from build123d import *

# Parameters (mm, degrees)
F1_DEPTH = 5


with BuildPart() as f1:
    # F0 (on Front) → F1 (new body)
    with BuildSketch(Plane.XZ):
        with BuildLine():
            ThreePointArc((0, -3), (2.12132, -2.12132), (3, 0))
            ThreePointArc((3, 0), (2.992298, 0.214837), (2.96923, 0.428571))
            ThreePointArc((2.96923, 0.428571), (0, 3), (-2.96923, 0.428571))
            ThreePointArc((-2.96923, 0.428571), (-2.267787, -1.963961), (0, -3))
        make_face()
        with BuildLine():
            ThreePointArc((-1.322876, -1.5), (-0.822876, 1.822876), (2, 0))
            ThreePointArc((2, 0), (1.822876, -0.822876), (1.322876, -1.5))
            ThreePointArc((1.322876, -1.5), (0, -2), (-1.322876, -1.5))
        make_face(mode=Mode.SUBTRACT)
        with BuildLine():
            ThreePointArc((2.96923, 0.428571), (2.992298, 0.214837), (3, 0))
            ThreePointArc((3, 0), (2.12132, -2.12132), (0, -3))
            ThreePointArc((0, -3), (2.618615, -3.976284), (3.958973, -6.428571))
            Line((3.958973, -6.428571), (2.96923, 0.428571))
        make_face()
        with BuildLine():
            ThreePointArc((-3.958973, -6.428571), (-2.618615, -3.976284), (0, -3))
            ThreePointArc((0, -3), (-2.267787, -1.963961), (-2.96923, 0.428571))
            Line((-2.96923, 0.428571), (-3.958973, -6.428571))
        make_face()
        with BuildLine():
            ThreePointArc((3.958973, -6.428571), (2.618615, -3.976284), (0, -3))
            ThreePointArc((0, -3), (-2.618615, -3.976284), (-3.958973, -6.428571))
            ThreePointArc((-3.958973, -6.428571), (-0.28645, -10.98973), (4, -7))
            ThreePointArc((4, -7), (3.98973, -6.71355), (3.958973, -6.428571))
        make_face()
        with BuildLine():
            ThreePointArc((2, -5.5), (2.371708, -6.209431), (2.5, -7))
            ThreePointArc((2.5, -7), (-0.790569, -9.371708), (-2, -5.5))
            ThreePointArc((-2, -5.5), (0, -4.5), (2, -5.5))
        make_face(mode=Mode.SUBTRACT)
        with BuildLine():
            Line((-2, -5.5), (2, -5.5))
            ThreePointArc((2, -5.5), (0, -4.5), (-2, -5.5))
        make_face()
        with BuildLine():
            Line((1.322876, -1.5), (-1.322876, -1.5))
            ThreePointArc((-1.322876, -1.5), (0, -2), (1.322876, -1.5))
        make_face()
    extrude(amount=F1_DEPTH)


solid = f1.part
Geometry check sheet. Reference: the model listing, model coordinates, mm. Give positions to 0.01 mm unless a question says otherwise; leave off trailing zeros. Loops run counter-clockwise (first coordinate to the right, second up) from the corner with the lowest first, then second, coordinate; pieces in that order, holes last.
(1) Thickness scan on L1, parallel to Z at x = 0, y = -1.5; L2, parallel to X at y = -1.55, z = -7; L3, parallel to Z at x = 1.75, y = -3.45. Record the ranges inside material, lowest first.
From the geometry:
L1: z = -11 to -9.5, -5.5 to -1.5, 2 to 3
L2: x = -4 to -2.5, 2.5 to 4
L3: z = -10.6 to -8.79, -5.5 to -0.97, 0.97 to 2.44
(2) Section check A-A on x = 0. Record the cut outline in (y, z), then the cut area to 3 significant figures.
From the geometry:
outline: (-5, -11) - (0, -11) - (0, -9.5) - (-5, -9.5) - close; (-5, -5.5) - (0, -5.5) - (0, -1.5) - (-5, -1.5) - close; (-5, 2) - (0, 2) - (0, 3) - (-5, 3) - close
area: 32.5 mm2
(3) Section check B-B on y = -1.7. Record the cut outline in (x, z).
From the geometry:
outline: (-3.96, -6.43) arc R4 ccw (long way) to (4, -7) arc R4 ccw to (3.96, -6.43) - (2.97, 0.43) arc R3 ccw to (-2.97, 0.43) - close; hole (-2, -5.5) arc R2.5 ccw (long way) to (2.5, -7) arc R2.5 ccw to (2, -5.5) - close; hole (-1.32, -1.5) - (1.32, -1.5) arc R2 ccw to (2, 0) arc R2 ccw (long way) to start
(4) Section check C-C on z = -6.25. Record the cut outline in (x, y).
From the geometry:
outline: (-3.93, -5) - (-2.38, -5) - (-2.38, 0) - (-3.93, 0) - close; (2.38, -5) - (3.93, -5) - (3.93, 0) - (2.38, 0) - close
(5) Depth check by flat-ended pin: pin 1 Ø0.8 at (x, y) = (0.5, -3) entering from +Z; pin 2 Ø1.5 at (x, y) = (-3, -3) entering from +Z; pin 3 Ø1.5 at (y, z) = (-1.5, -1.5) entering from -X. Enter the tip coordinate at first touch or a pass-through.
From the geometry:
pin 1: stops at z = 3
pin 2: stops at z = 1.98
pin 3: stops at x = -3.36
(6) Section check D-D on z = -8. Record the cut outline in (x, y), then the cut area to 3 significant figures.
From the geometry:
outline: (-3.87, -5) - (-2.29, -5) - (-2.29, 0) - (-3.87, 0) - close; (2.29, -5) - (3.87, -5) - (3.87, 0) - (2.29, 0) - close
area: 15.8 mm2
(7) Release check for a two-part mould opening along X. For faces 1 (the flat face through (0, -2, -1.5)), 2 (the flat face through (0, 0, -4)), 3 (the flat face through (3.47, -2.46, -3.05)), 4 (the flat face through (0, -2, -5.5)) record: released by +X, released by -X, zero draft, split by the parting line, or undercut.
From the geometry:
face 1: undercut
face 2: zero draft
face 3: released by +X
face 4: undercut
